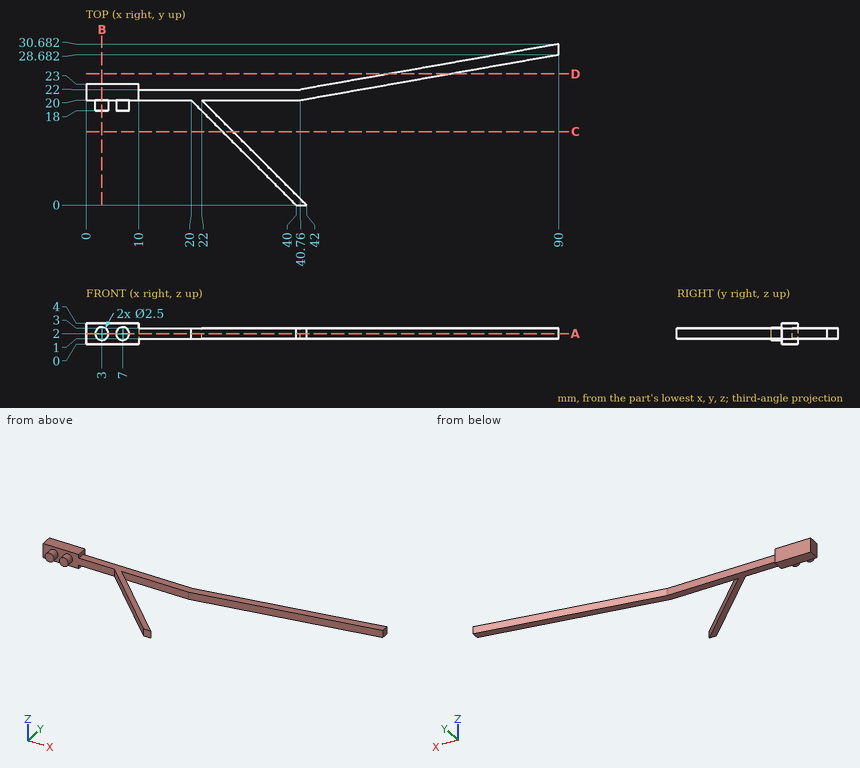
Job drawing, mm, ordinate dimensions from the low corner. One solid piece. Give positions to 0.01 mm unless a question says otherwise; leave off trailing zeros. Order: outer loops, then holes, each group sorted by start corner. A loop starts at its lowest first (then second) coordinate and runs counter-clockwise, first axis right, second up. Notation, with made-up numbers: (-0.75, 7.25) - (32.25, 7.25) arc R20 cw to (32.25, 23.25) - close; hole circle Ø8 at (29, 38.5). An arc over 180 degrees is marked (long way). Return JSON: item names as keys, results as strings.
1) Probe line 1 (Y direction, x = 17, z = 2.3); line 2 (Z direction, x = 45.5, y = 21); line 3 (Y direction, x = 39, z = 1.65). List the from-to ranges inside material, lowest first. Write a range as from..to.
Geometry says:
{"line 1": "20..22", "line 2": "1..3", "line 3": "1..3, 20..22"}
2) Cut at D-D, the plane y = 25. Give the cut face in (x, z), plus the area to 3 significant figures.
Geometry says:
{"outline": "(57.77, 1) - (69.12, 1) - (69.12, 3) - (57.77, 3) - close", "area": "22.7 mm²"}
3) Cut at A-A, the plane z = 2. Give the cut face in (x, y), plus the area to 3 significant figures.
Geometry says:
{"outline": "(0, 20) - (1.75, 20) - (1.75, 18) - (4.25, 18) - (4.25, 20) - (5.75, 20) - (5.75, 18) - (8.25, 18) - (8.25, 20) - (20, 20) - (40, 0) - (42, 0) - (22, 20) - (40.76, 20) - (90, 28.68) - (90, 30.68) - (40.76, 22) - (10, 22) - (10, 23) - (0, 23) - close", "area": "240 mm²"}
4) Cut at C-C, the plane y = 14. Give the cut face in (x, z).
Geometry says:
{"outline": "(26, 1) - (28, 1) - (28, 3) - (26, 3) - close"}
5) Cut at B-B, the plane x = 3. Give the cut face in (y, z), plus the area to 3 significant figures.
Geometry says:
{"outline": "(18, 0.75) - (20, 0.75) - (20, 0) - (23, 0) - (23, 4) - (20, 4) - (20, 3.25) - (18, 3.25) - close", "area": "17.0 mm²"}
6) Flat gauge pins, fed straight in: P1, Ø2, axis at x = 58, z = 2, coming from the -Y side; P2, Ø1.5, axis at y = 11, z = 2, coming from the -X side; P3, Ø1.2, axis at x = 13.5, z = 1.5, coming from the -Y side. Where does each tip first touch, or does it go through?
Geometry says:
{"P1": "y = 22.86", "P2": "x = 28.25", "P3": "y = 20"}
